from build123d import *

# Parameters (mm, degrees)
F1_DEPTH = 3


with BuildPart() as f1:
    # F0 (on Front) → F1 (new body)
    with BuildSketch(Plane.XZ):
        with BuildLine():
            ThreePointArc((-37.269928, 56.85529), (-44.340996, 53.926358), (-47.269928, 46.85529))
            Line((-47.269928, 46.85529), (-47.269928, 1.85529))
            Line((-47.269928, 1.85529), (-47.269928, -43.14471))
            ThreePointArc((-47.269928, -43.14471), (-44.340996, -50.215777), (-37.269928, -53.14471))
            Line((-37.269928, -53.14471), (-25.093389, -53.14471))
            Line((-25.093389, -53.14471), (-12.269928, -25.64471))
            Line((-12.269928, -25.64471), (-12.269928, -20.64471))
            Line((-12.269928, -20.64471), (-18.269928, -20.64471))
            Line((-18.269928, -20.64471), (-18.269928, -17.64471))
            Line((-18.269928, -17.64471), (-12.269928, -17.64471))
            Line((-12.269928, -17.64471), (-12.269928, 1.85529))
            Line((-12.269928, 1.85529), (-12.269928, 21.35529))
            Line((-12.269928, 21.35529), (-18.269928, 21.35529))
            Line((-18.269928, 21.35529), (-18.269928, 24.35529))
            Line((-18.269928, 24.35529), (-12.269928, 24.35529))
            Line((-12.269928, 24.35529), (-12.269928, 29.35529))
            Line((-12.269928, 29.35529), (-25.093389, 56.85529))
            Line((-25.093389, 56.85529), (-37.269928, 56.85529))
        make_face()
        with BuildLine():
            ThreePointArc((-42.769928, 43.85529), (-41.891248, 45.976611), (-39.769928, 46.85529))
            Line((-39.769928, 46.85529), (-30.769928, 46.85529))
            ThreePointArc((-30.769928, 46.85529), (-28.648608, 45.976611), (-27.769928, 43.85529))
            Line((-27.769928, 43.85529), (-27.769928, 1.85529))
            Line((-27.769928, 1.85529), (-27.769928, -40.14471))
            ThreePointArc((-27.769928, -40.14471), (-28.648608, -42.26603), (-30.769928, -43.14471))
            Line((-30.769928, -43.14471), (-39.769928, -43.14471))
            ThreePointArc((-39.769928, -43.14471), (-41.891248, -42.26603), (-42.769928, -40.14471))
            Line((-42.769928, -40.14471), (-42.769928, 1.85529))
            Line((-42.769928, 1.85529), (-42.769928, 43.85529))
        make_face(mode=Mode.SUBTRACT)
    extrude(amount=F1_DEPTH)


solid = f1.part
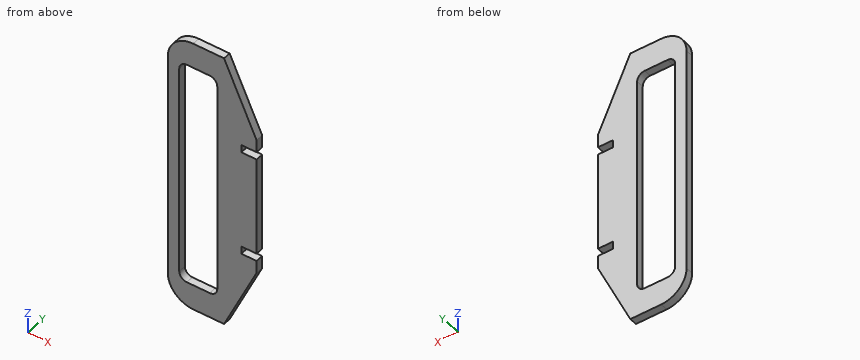
Source: CAD feature listing. Evaluate the final solid. Frame: model axes, mm. Round coordinates to 2 decimals unless told otherwise and drop trailing zeros. Order: outer loops, then holes, each group sorted by start corner. A loop starts at its lowest first (then second) coordinate and runs counter-clockwise, first axis right, second up. Notation, with made-up numbers: (19, -4) - (33, -4) arc R30 ccw to (33, 21) - close; hole circle Ø3 at (-15, -38). An arc over 180 degrees is marked (long way). Use a Markdown table: item, result. Add a question column.
1. First-contact query: pin 1 (1.5 mm diameter, centred on x = -22.5, z = -34, fed in from +Y); pin 2 (1.5 mm diameter, centred on y = -1.5, z = 23.5, fed in from +X); pin 3 (1.5 mm diameter, centred on x = -16, y = -1, fed in from +Z); pin 4 (0.9 mm diameter, centred on x = -15.5, y = -1, fed in from -Z). Flat tips, straight axial feed; report the tip coordinate or a pass-through.
2. Section query D-D (x = -14.5). Return the cut outline in (y, z).
3. Section query A-A (x = -35). Return the cut outline in (y, z), then the cut area to 3 significant figures.
4. Line query: probe 1 along X at (y, z) = (-1.7, 21); probe 2 along Z at (x, y) = (-32, -2.5); probe 3 along X at (y, z) = (-1.9, -18). Output: solid intervals per line, ascending.
5. Section query B-B (z = 9.5). Return the cut outline in (x, y).
6. Section query C-C (y = -2.5). Return the cut outline in (x, z), then the cut area to 3 significant figures.
Derived:
| question | item | result |
|---|---|---|
| 1 | pin 1 | y = 0 |
| 1 | pin 2 | x = -18.27 |
| 1 | pin 3 | z = 38.96 |
| 1 | pin 4 | z = -33.54 |
| 2 | outline | (-3, -30.43) - (0, -30.43) - (0, -20.64) - (-3, -20.64) - close; (-3, -17.64) - (0, -17.64) - (0, 21.36) - (-3, 21.36) - close; (-3, 24.36) - (0, 24.36) - (0, 34.14) - (-3, 34.14) - close |
| 3 | outline | (-3, -53.14) - (0, -53.14) - (0, -43.14) - (-3, -43.14) - close; (-3, 46.86) - (0, 46.86) - (0, 56.86) - (-3, 56.86) - close |
| 3 | area | 60.0 mm2 |
| 4 | probe 1 | -47.27 to -42.77, -27.77 to -12.27 |
| 4 | probe 2 | -53.14 to -43.14, 46.86 to 56.86 |
| 4 | probe 3 | -47.27 to -42.77, -27.77 to -18.27 |
| 5 | outline | (-47.27, -3) - (-42.77, -3) - (-42.77, 0) - (-47.27, 0) - close; (-27.77, -3) - (-12.27, -3) - (-12.27, 0) - (-27.77, 0) - close |
| 6 | outline | (-47.27, -43.14) arc R10 ccw to (-37.27, -53.14) - (-25.09, -53.14) - (-12.27, -25.64) - (-12.27, -20.64) - (-18.27, -20.64) - (-18.27, -17.64) - (-12.27, -17.64) - (-12.27, 21.36) - (-18.27, 21.36) - (-18.27, 24.36) - (-12.27, 24.36) - (-12.27, 29.36) - (-25.09, 56.86) - (-37.27, 56.86) arc R10 ccw to (-47.27, 46.86) - close; hole (-42.77, -40.14) arc R3 ccw to (-39.77, -43.14) - (-30.77, -43.14) arc R3 ccw to (-27.77, -40.14) - (-27.77, 43.86) arc R3 ccw to (-30.77, 46.86) - (-39.77, 46.86) arc R3 ccw to (-42.77, 43.86) - close |
| 6 | area | 2,080 mm2 |
